Could you check a few things on this drawing? It's one solid part, dimensions in mm from its lowest x, y, z. Round coordinates to 2 decimals unless told otherwise and drop trailing zeros. Write each loop counter-clockwise with the first axis right and the second up, starting at its lowest first coordinate (ties: lowest second). Pieces come first, ordered by that corner, then holes. Notation, with made-up numbers: (-35, 1.25) -> (-22, 1.25) arc R17 ccw to (-22, 10.25) -> close; hole circle Ø8 at (33, 16). An arc over 180 degrees is marked (long way). Answer in a Markdown table with one row per item. Add a question column.
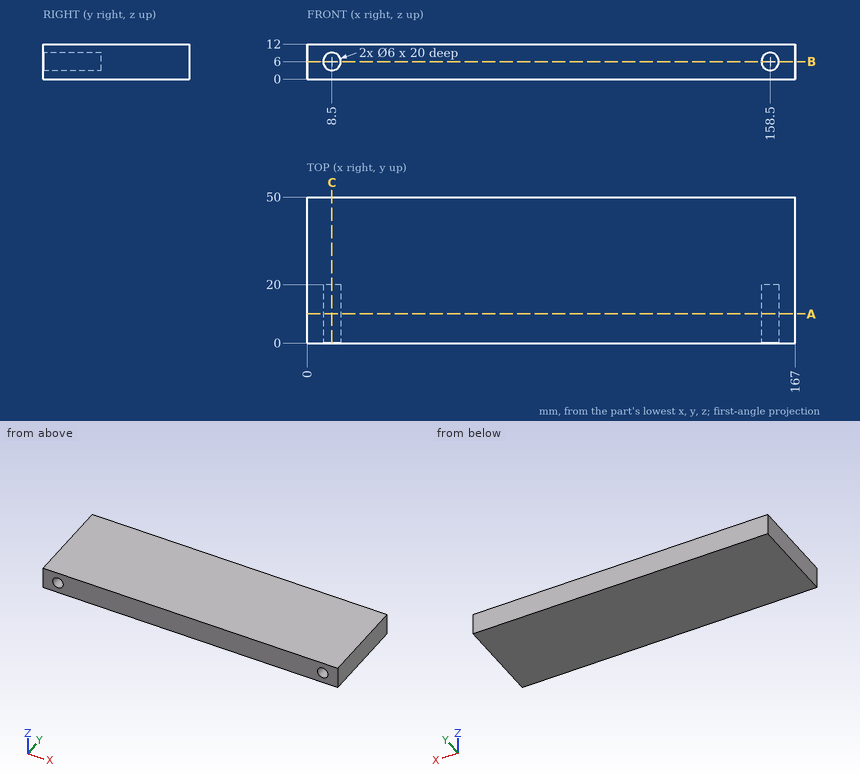
(1) I need wall thicknesses on L1, parallel to X at y = 13.75, z = 6; L2, parallel to Z at x = 158.5, y = 8; L3, parallel to X at y = 6, z = 7. Which ranges of each line are inside material? Lowest first, please.
(2) Suppose I cut it at A-A, the plane y = 10. Please give me the cut outline in (x, z).
(3) Suppose I cut it at B-B, the plane z = 6. Please give me the cut outline in (x, y).
(4) Suppose I cut it at C-C, the plane x = 8.5. Please give me the cut outline in (y, z).
Response:
| question | item | result |
|---|---|---|
| 1 | L1 | 0 to 5.5, 11.5 to 155.5, 161.5 to 167 |
| 1 | L2 | 0 to 3, 9 to 12 |
| 1 | L3 | 0 to 5.67, 11.33 to 155.67, 161.33 to 167 |
| 2 | outline | (0, 0) -> (167, 0) -> (167, 12) -> (0, 12) -> close; hole circle Ø6 at (8.5, 6); hole circle Ø6 at (158.5, 6) |
| 3 | outline | (0, 0) -> (5.5, 0) -> (5.5, 20) -> (11.5, 20) -> (11.5, 0) -> (155.5, 0) -> (155.5, 20) -> (161.5, 20) -> (161.5, 0) -> (167, 0) -> (167, 50) -> (0, 50) -> close |
| 4 | outline | (0, 0) -> (50, 0) -> (50, 12) -> (0, 12) -> (0, 9) -> (20, 9) -> (20, 3) -> (0, 3) -> close |
